```python
from build123d import *

# Parameters (mm, degrees)
F0_W     = 200
F0_H     = 20
F1_DEPTH = 1
F3_D     = 5
F4_R     = 2.5


with BuildPart() as f1:
    # F0 (on Top) → F1 (new body)
    with BuildSketch(Plane.XY):
        with Locations((100, 10)):
            Rectangle(F0_W, F0_H)
    extrude(amount=F1_DEPTH)

    # F3 (through all)
    with Locations(Plane.XY.offset(1)):
        with Locations((10, 10)):
            Hole(F3_D / 2)

    # F4
    f4_edges = [f1.edges().sort_by_distance(p)[0] for p in [
        (0, 20, 0.5),
        (0, 0, 0.5),
        (200, 0, 0.5),
        (200, 20, 0.5),
    ]]
    fillet(f4_edges, radius=F4_R)


solid = f1.part
```
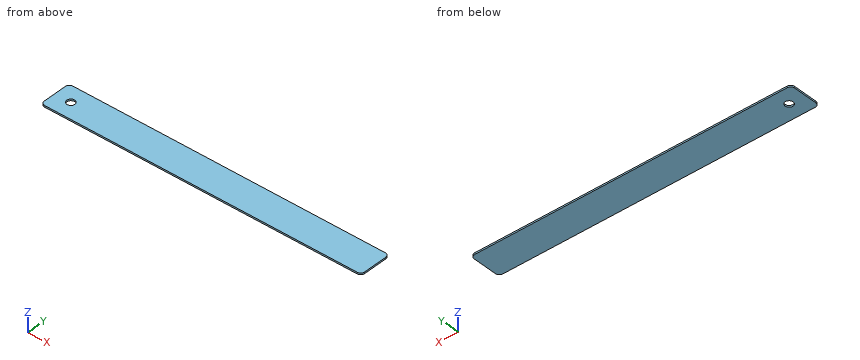
Verification items for the finished model (mm, model axes). Round coordinates to 2 decimals unless told otherwise and drop trailing zeros. Order: outer loops, then holes, each group sorted by start corner. A loop starts at its lowest first (then second) coordinate and runs counter-clockwise, first axis right, second up. Notation, with made-up numbers: (-33.5, 67.25) - (12.5, 67.25) arc R16 ccw to (12.5, 98.25) - close; hole circle Ø1 at (16.5, 70). An arc over 180 degrees is marked (long way). Use CSV: the item, a comma, the result in double quotes.
(1) Section check A-A on x = 10. Record the boundary of the cut face in (y, z).
Entries:
outline,"(0, 0) - (7.5, 0) - (7.5, 1) - (0, 1) - close; (12.5, 0) - (20, 0) - (20, 1) - (12.5, 1) - close"
(2) Section check B-B on y = 10. Record the boundary of the cut face in (x, z), and give its area (3 significant figures).
Entries:
outline,"(0, 0) - (7.5, 0) - (7.5, 1) - (0, 1) - close; (12.5, 0) - (200, 0) - (200, 1) - (12.5, 1) - close"
area,"195 mm^2"
(3) Thickness scan on probe 1 along X at (y, z) = (9.75, 0.35); probe 2 along X at (y, z) = (8.5, 0.9); probe 3 along X at (y, z) = (18.5, 0.15). Record the ranges inside material, lowest first. Write a range as from..to.
Entries:
probe 1,"0..7.51, 12.49..200"
probe 2,"0..8, 12..200"
probe 3,"0.21..199.79"
